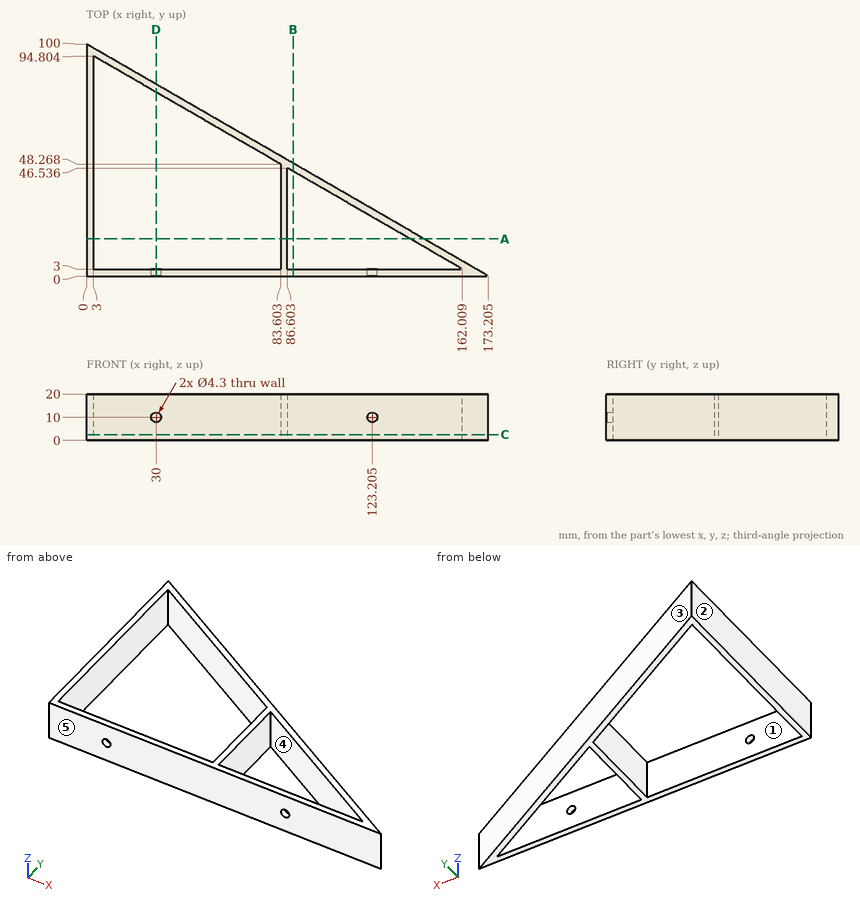
Geometry: see drawing. Coordinates: mm, zero at the bounding-box minimum. A direction names the side the tool comes from. Round coordinates to 2 decimals unless told otherwise and drop trailing zeros. Loops run counter-clockwise (first coordinate to the right, second up) from the corner with the lowest first, then second, coordinate; pieces in that order, holes last.
(1) Material intervals for probe 1 along Z at (x, y) = (30, 1); probe 2 along X at (y, z) = (73.5, 18.75); probe 3 along Y at (x, z) = (49, 9.75) (1 decimal), sorted ascending.
From the geometry:
probe 1: z = 0 to 7.85, 12.15 to 20
probe 2: x = 0 to 3, 39.9 to 45.9
probe 3: y = 0 to 3, 68.2 to 71.7
(2) Access query for the marked faces 4 and 5. Directions: +Z, -Z, +X, -X, +Y, -Y. A direction counts if a zero-diameter tool reaches every point of the face in a straight line with its end or side. Return the directions, or none.
From the geometry:
face 4: +Z, -Z
face 5: +Z, -Z, +X, -X, -Y
(3) Contact query for flat-ended pins moving along their axis: pin 1 Ø4 at (x, z) = (137.5, 11) entering from +Y; pin 2 Ø8 at (y, z) = (36.5, 5) entering from +X (1 decimal); pin 3 Ø8 at (y, z) = (17.5, 15) entering from +X (1 decimal). Output: stop coordinate, or through.
From the geometry:
pin 1: stops at y = 21.77
pin 2: stops at x = 116.9
pin 3: stops at x = 149.8
(4) Section query B-B (x = 89). Output: boundary loops of the cut face in (y, z) (1 decimal).
From the geometry:
outline: (0, 0) - (3, 0) - (3, 20) - (0, 20) - close; (45.2, 0) - (48.6, 0) - (48.6, 20) - (45.2, 20) - close
(5) Pull-direction query (X, two-part tool) for the marked faces 1, 2 and 3; classes: +X half, -X half, draft (parallel to the pull), parting line (faces both ways), or undercut.
From the geometry:
face 1: undercut
face 2: -X half
face 3: +X half
(6) Section query D-D (x = 30). Give the number of separate pieces and of enclosed holes in the cut face, and give its area (3 significant figures).
From the geometry:
separate pieces: 3
enclosed holes: 0
area: 116 mm2
(7) Section query C-C (z = 2.5). Output: boundary loops of the cut face in (x, y) (1 decimal).
From the geometry:
outline: (0, 0) - (173.2, 0) - (0, 100) - close; hole (3, 3) - (83.6, 3) - (83.6, 48.3) - (3, 94.8) - close; hole (86.6, 3) - (162, 3) - (86.6, 46.5) - close
(8) Section query A-A (y = 16). Output: boundary loops of the cut face in (x, z), and give its area (3 significant figures).
From the geometry:
outline: (0, 0) - (3, 0) - (3, 20) - (0, 20) - close; (83.6, 0) - (86.6, 0) - (86.6, 20) - (83.6, 20) - close; (139.49, 0) - (145.49, 0) - (145.49, 20) - (139.49, 20) - close
area: 240 mm2
